Model file for the job. Use its own axes, mm. A direction names the side the tool comes from. Coordinates: 2 decimals unless noted, no trailing zeros. Loops run counter-clockwise (first coordinate to the right, second up) from the corner with the lowest first, then second, coordinate; pieces in that order, holes last. Notation, with made-up numbers: (-2, 87.5) - (39, 87.5) arc R22 ccw to (39, 97.5) - close; hole circle Ø2 at (57, -27.75). An arc over 180 degrees is marked (long way). Write each question's results on one line, items separated by ' | '. Start each with the question number.
```python
from build123d import *

# Parameters (mm, degrees)
F2_R = 2.54


with BuildPart() as f1:
    # F0 (on Right) → F1 (revolve)
    with BuildSketch(Plane.YZ):
        Polygon((-3.175, 0), (0, 0), (0, 57.15), (12.7, 57.15), (12.7, 89.419909), (47.625, 89.419909), (47.625, 101.6), (44.45, 101.6), (44.45, 92.594909), (-44.45, 92.594909), (-44.45, 101.6), (-47.625, 101.6), (-47.625, 89.419909), (9.525, 89.419909), (9.525, 60.325), (-3.175, 60.325), align=None)
    revolve(axis=Axis((0, -1.5875, 0), (0, 1, 0)))

    # F2
    f2_edges = [f1.edges().sort_by_distance(p)[0] for p in [
        (0, -47.625, -101.6),
        (0, -47.625, -89.419909),
        (0, 9.525, -89.419909),
        (0, 9.525, -60.325),
        (0, -3.175, -60.325),
    ]]
    fillet(f2_edges, radius=F2_R)


solid = f1.part
```
Q1. Drill centre lines: L1, parallel to X at y = -26, z = 0; L2, parallel to Y at x = 33.5, z = -87.5 (3 decimals); L3, parallel to Z at x = -25, y = -2. Where is each one in solid material? Low to high. Write a range as from..to.
Q2. Cut at A-A (y = 25). List the corners of the cut face in (x, z).
Q3. Which spindle directions (+Z, -Z, +X, -X, +Y, -Y) get a long thin tool onto all of the face, cutting with end or side? Do faces 4 (the cylindrical face through (-90.393, -0.622, -20.073)), 5 (the cylindrical face through (-87.294, -18.686, -19.384)), 6 (the cylindrical face through (2.513, 6.439, -57.095)), 7 (the flat face through (-90, 47.625, 0)). Say none if no direction does.
Q4. Mould opens along X. For faces 1 (the flat face through (1, 0, 1)), 2 (the flat face through (-90, 44.45, -23)), 3 (the cylindrical face through (-99.184, 46.015, -22.025)) say: +X half, -X half, draft (parallel to the pull), parting line (faces both ways), or undercut.
Q5. Pin check, flat tips, straight feed: pin 1 (2 mm diameter, centred on x = 6, y = 9, fed in from -Z); pin 2 (1.5 mm diameter, centred on x = 31.5, z = 35, fed in from -Y) (3 decimals); pin 3 (3 mm diameter, centred on x = -13.5, y = -4, fed in from +Z). Stop position of each tip, or through.
Check result:
1) L1: -92.59..-89.42, 89.42..92.59 | L2: -47.625..-44.45, 44.45..47.625 | L3: -89.16..-85.85, -54.46..54.46, 85.85..89.16
2) outline: circle Ø185.19 at (0, 0); hole circle Ø178.84 at (0, 0)
3) face 4: none | face 5: -Y | face 6: +Y | face 7: +Z, -Z, +X, -X, +Y
4) face 1: undercut | face 2: draft | face 3: parting line
5) pin 1: z = -92.46 | pin 2: y = -3.175 | pin 3: z = 91.81
